Source: three-view drawing plus pictorial views. Frame: mm from the lowest corner of the part. Round coordinates to 2 decimals unless told otherwise and drop trailing zeros. Loops run counter-clockwise (first coordinate to the right, second up) from the corner with the lowest first, then second, coordinate; pieces in that order, holes last. Notation, with made-up numbers: M 54,0.5 L 96,0.5 A27 ccw 96,37.5 Z; hole C -0.5,-40 d3. An arc over 180 degrees is marked long. Return JSON: item names as keys, results as strings. Group by question number.
1) Section C-C (z = 5). Output: boundary loops of the cut face in (x, y), plus the area to 3 significant figures.
2) Section A-A (x = 15). Output: boundary loops of the cut face in (y, z), plus the area to 3 significant figures.
3) Material intervals for line 1 (Y direction, x = 15, z = 5); line 2 (X direction, y = 19, z = 3); line 3 (Y direction, x = 15.5, z = 2.75), sorted ascending. Write a range as from..to.
4) Contact query for flat-ended pins moving along their axis: P1, Ø2, axis at y = 19.5, z = 1.5, coming from the -X side; P2, Ø2, axis at y = 21, z = 3.5, coming from the +X side; P3, Ø1.5, axis at x = 12, z = 4.5, coming from the +Y side. Output: stop coordinate, or through.
5) Mould query, pull axis X, two halves, no side actions, for the marked faces 1, 2 and 3. Classes: +X half, -X half, draft (parallel to the pull), parting line (faces both ways), or undercut.
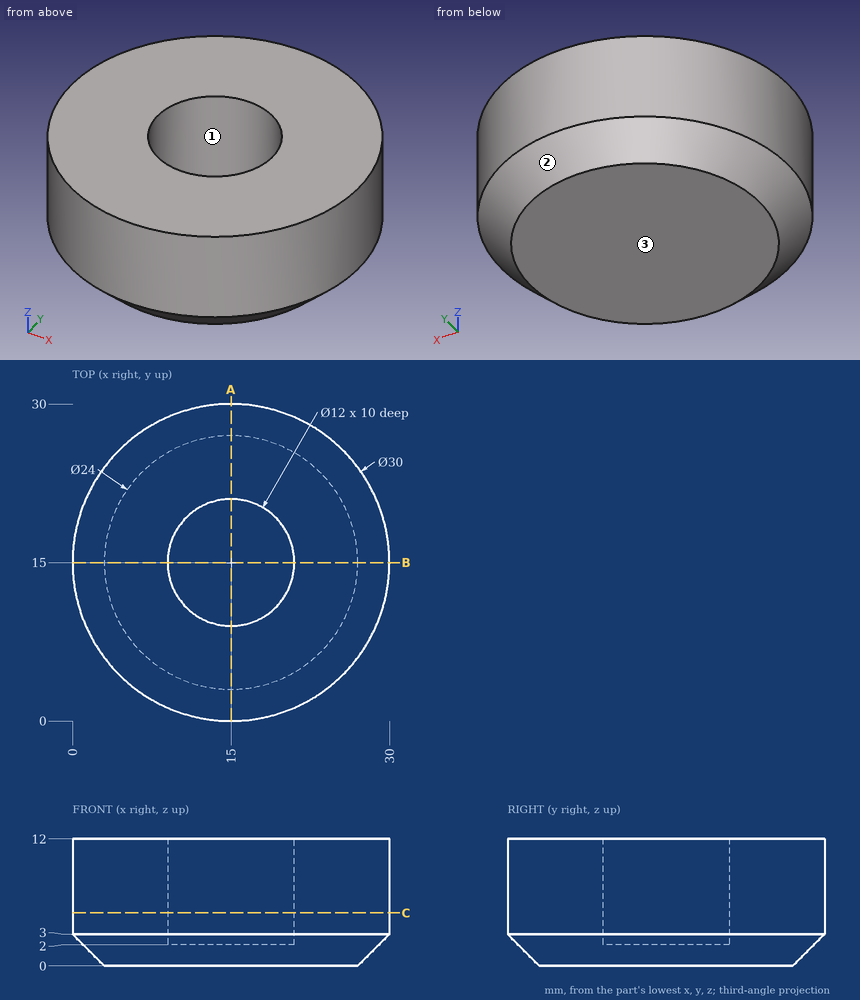
Returned:
{
 "1": {"outline": "C 15,15 d30; hole C 15,15 d12", "area": "594 mm^2"},
 "2": {"outline": "M 0,3 L 3,0 L 27,0 L 30,3 L 30,12 L 21,12 L 21,2 L 9,2 L 9,12 L 0,12 Z", "area": "231 mm^2"},
 "3": {"line 1": "y = 0..9, 21..30", "line 2": "x = 0.54..10.53, 19.47..29.46", "line 3": "y = 0.26..9.02, 20.98..29.74"},
 "4": {"P1": "stops at x = 1.17", "P2": "stops at x = 29.14", "P3": "stops at y = 29.83"},
 "5": {"face 1": "undercut", "face 2": "parting line", "face 3": "draft"}
}
